For this review, use the dimensioned drawing (mm, ordinates from the lowest corner) and the shaded views. A direction names the side the tool comes from. Coordinates: 2 decimals unless noted, no trailing zeros. Loops run counter-clockwise (first coordinate to the right, second up) from the corner with the lowest first, then second, coordinate; pieces in that order, holes last. Notation, with made-up numbers: (52, -32) - (89, -32) arc R17 cw to (89, -16) - close; hole circle Ø6 at (54, -35.75). An arc over 180 degrees is marked (long way). Use a Markdown table: item, result. Add a question column.
1) Add section A-A, the plane y = 28.5. Give the boundary of the cut face in (x, z), and give its area (3 significant figures).
2) For the marked faces 1, 2, 3, 4 and 5, list the 3-axis set-ups (+Z, -Z, +X, -X, +Y, -Y) from which the entire face can be reached by the end or side of a thin tool; tool diameter is ignored.
3) Add section C-C, the plane x = 116.5. Give the boundary of the cut face in (y, z).
4) Add section B-B, the plane z = 40. Give the boundary of the cut face in (x, y), and give its area (3 significant figures).
5) The part is to be moulded in two halves that separate along X. For the marked faces 6, 7 and 8, say which applies: pulls with the +X half, pulls with the -X half, needs draft (parallel to the pull), parting line crosses it, or undercut.
6) To check wall thickness, follow L1, parallel to X at y = 50.75, z = 35.75 (1 decimal); L2, parallel to X at y = 17, z = 52.5; L3, parallel to X at y = 52.35, z = 12.5. State the ranges of each line that lie inside material, in increasing order. Write a range as [from, to].
7) Clearance check with flat-ended pins moving along their axes: pin 1 (10 mm diameter, centred on y = 28, z = 22, fed in from +X); pin 2 (9 mm diameter, centred on x = 12.5, z = 21.5, fed in from +Y); pin 3 (12 mm diameter, centred on x = 43, z = 53.5, fed in from -Y). State where each tip first meets the part, or that it passes through.
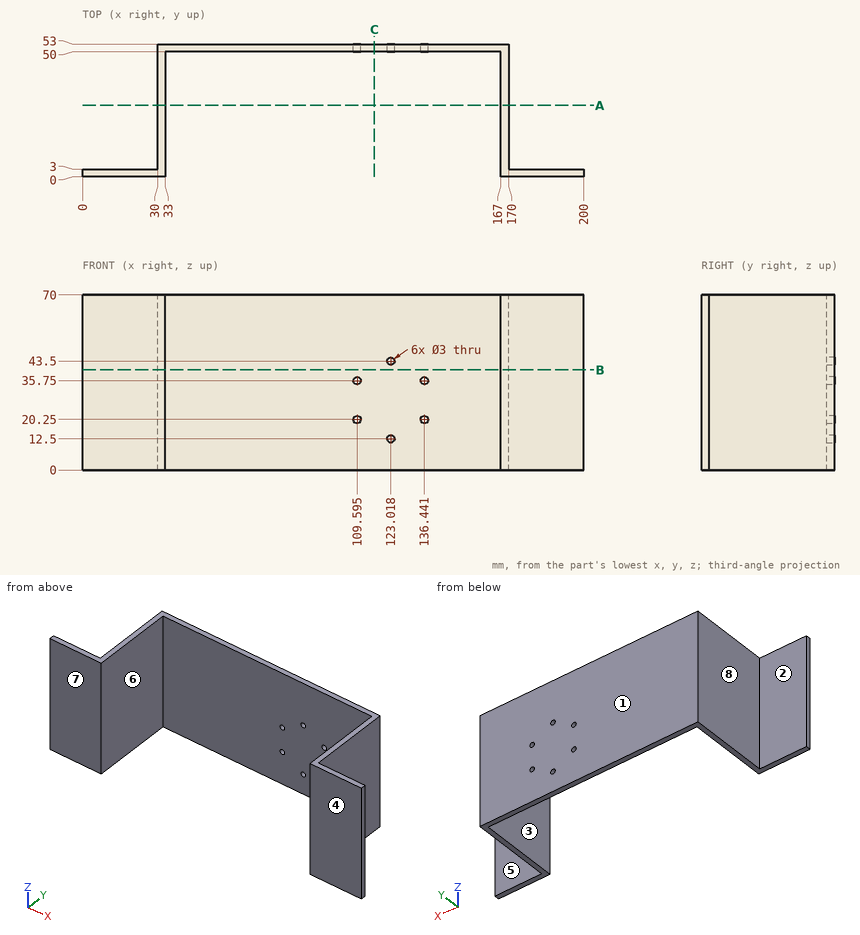
From the geometry:
| question | item | result |
|---|---|---|
| 1 | outline | (30, 0) - (33, 0) - (33, 70) - (30, 70) - close; (167, 0) - (170, 0) - (170, 70) - (167, 70) - close |
| 1 | area | 420 mm^2 |
| 2 | face 1 | +Z, -Z, +X, -X, +Y |
| 2 | face 2 | +Z, -Z, -X, +Y |
| 2 | face 3 | +Z, -Z, -Y |
| 2 | face 4 | +Z, -Z, +X, -X, -Y |
| 2 | face 5 | +Z, -Z, +X, +Y |
| 3 | outline | (50, 0) - (53, 0) - (53, 70) - (50, 70) - close |
| 4 | outline | (0, 0) - (33, 0) - (33, 50) - (167, 50) - (167, 0) - (200, 0) - (200, 3) - (170, 3) - (170, 53) - (30, 53) - (30, 3) - (0, 3) - close |
| 4 | area | 900 mm^2 |
| 5 | face 6 | undercut |
| 5 | face 7 | needs draft |
| 5 | face 8 | pulls with the -X half |
| 6 | L1 | x = [30, 108.1], [111.1, 134.9], [137.9, 170] |
| 6 | L2 | x = [30, 33], [167, 170] |
| 6 | L3 | x = [30, 121.52], [124.52, 170] |
| 7 | pin 1 | stops at x = 170 |
| 7 | pin 2 | stops at y = 3 |
| 7 | pin 3 | stops at y = 50 |
